Part model, mm, in its own coordinate system. A direction names the side the tool comes from. Give positions to 0.01 mm unless a question says otherwise; leave off trailing zeros. Write each loop counter-clockwise with the first axis right and the second up, starting at its lowest first coordinate (ties: lowest second). Pieces come first, ordered by that corner, then holes. Notation, with made-up numbers: M -7.75,8.25 L 25.25,8.25 A33 cw 25.25,47.25 Z; hole C 85,86.25 d2. An arc over 180 degrees is marked long. Answer as CSV lines item,"result". Start each with the question number.
1) Pin check, flat tips, straight feed: pin 1 Ø4 at (y, z) = (-3.5, -1.5) entering from -X; pin 2 Ø5 at (x, z) = (6.5, -7.5) entering from -Y; pin 3 Ø2 at (x, z) = (9, 8.5) entering from -Y. Stop position of each tip, or through.
2) Slice it at A-A, the plane y = 0. Give the cut face in (x, z), plus the area to 3 significant figures.
3) Slice it at B-B, the plane x = 0. Give the cut face in (y, z).
4) Wall check: line 1 along Y through (x, z) = (0, 2); line 2 along Y through (x, z) = (-0.75, 4); line 3 along X through (y, z) = (-6.25, -12.5). Give the ranges that are in metal, low to high. Write a range as from..to.
5) Mould opens along X. For faces 3 (the cylindrical face through (-11.34, 6.56, 0.22)), 4 (the cylindrical face through (-6.29, 10.918, 0.217)), 5 (the cylindrical face through (7.7, -10.6, 0.2)) say: pulls with the +X half, pulls with the -X half, needs draft (parallel to the pull), parting line crosses it, or undercut.
6) Tool access for faces 1 (the cylindrical face through (-2.73, -12.812, 0.217)), 2 (the cylindrical face through (8.44, 9.356, 0.217)): list every direction of +Z, -Z, +X, -X, +Y, -Y with a clear straight run to the whole face (end or side of a thin tool).
```python
from build123d import *

# Parameters (mm, degrees)
F0_R     = 12.5
F1_DEPTH = 15.5
F0_R_2   = 11.1
F2_DEPTH = 15.5


with BuildPart() as f1:
    # F0 (on Top) → F1 (new body, symmetric)
    with BuildSketch(Plane.XY):
        with BuildLine():
            Line((0.5, -13.090455), (0.480916, -12.590819))
            ThreePointArc((0.480916, -12.590819), (1.317059, -12.530976), (2.147372, -12.415667))
            Line((2.147372, -12.415667), (2.232585, -12.908353))
            ThreePointArc((2.232585, -12.908353), (2.723643, -12.813734), (3.210732, -12.700441))
            Line((3.210732, -12.700441), (3.088185, -12.215691))
            ThreePointArc((3.088185, -12.215691), (3.893614, -11.983312), (4.681809, -11.697892))
            Line((4.681809, -11.697892), (4.867595, -12.162094))
            ThreePointArc((4.867595, -12.162094), (5.32825, -11.967445), (5.78114, -11.755357))
            Line((5.78114, -11.755357), (5.560486, -11.306679))
            ThreePointArc((5.560486, -11.306679), (6.3, -10.91192), (7.011628, -10.468862))
            Line((7.011628, -10.468862), (7.289868, -10.884293))
            ThreePointArc((7.289868, -10.884293), (7.699987, -10.598123), (8.098885, -10.296508))
            Line((8.098885, -10.296508), (7.789767, -9.903511))
            ThreePointArc((7.789767, -9.903511), (8.431046, -9.363625), (9.035006, -8.782293))
            Line((9.035006, -8.782293), (9.393538, -9.130796))
            ThreePointArc((9.393538, -9.130796), (9.735197, -8.765611), (10.062669, -8.387651))
            Line((10.062669, -8.387651), (9.678598, -8.067512))
            ThreePointArc((9.678598, -8.067512), (10.193614, -7.406094), (10.663511, -6.711895))
            Line((10.663511, -6.711895), (11.086666, -6.97824))
            ThreePointArc((11.086666, -6.97824), (11.344933, -6.55), (11.586666, -6.112215))
            Line((11.586666, -6.112215), (11.144427, -5.878924))
            ThreePointArc((11.144427, -5.878924), (11.510673, -5.124882), (11.825969, -4.348155))
            Line((11.825969, -4.348155), (12.295254, -4.520701))
            ThreePointArc((12.295254, -4.520701), (12.45884, -4.048123), (12.604271, -3.569645))
            Line((12.604271, -3.569645), (12.123192, -3.433399))
            ThreePointArc((12.123192, -3.433399), (12.32466, -2.619687), (12.471576, -1.79438))
            Line((12.471576, -1.79438), (12.966479, -1.865586))
            ThreePointArc((12.966479, -1.865586), (13.028237, -1.369323), (13.071008, -0.871064))
            Line((13.071008, -0.871064), (12.572114, -0.837817))
            ThreePointArc((12.572114, -0.837817), (12.6, 0), (12.572114, 0.837817))
            Line((12.572114, 0.837817), (13.071008, 0.871064))
            ThreePointArc((13.071008, 0.871064), (13.028237, 1.369323), (12.966479, 1.865586))
            Line((12.966479, 1.865586), (12.471576, 1.79438))
            ThreePointArc((12.471576, 1.79438), (12.32466, 2.619687), (12.123192, 3.433399))
            Line((12.123192, 3.433399), (12.604271, 3.569645))
            ThreePointArc((12.604271, 3.569645), (12.45884, 4.048123), (12.295254, 4.520701))
            Line((12.295254, 4.520701), (11.825969, 4.348155))
            ThreePointArc((11.825969, 4.348155), (11.510673, 5.124882), (11.144427, 5.878924))
            Line((11.144427, 5.878924), (11.586666, 6.112215))
            ThreePointArc((11.586666, 6.112215), (11.344933, 6.55), (11.086666, 6.97824))
            Line((11.086666, 6.97824), (10.663511, 6.711895))
            ThreePointArc((10.663511, 6.711895), (10.193614, 7.406094), (9.678598, 8.067512))
            Line((9.678598, 8.067512), (10.062669, 8.387651))
            ThreePointArc((10.062669, 8.387651), (9.735197, 8.765611), (9.393538, 9.130796))
            Line((9.393538, 9.130796), (9.035006, 8.782293))
            ThreePointArc((9.035006, 8.782293), (8.431046, 9.363625), (7.789767, 9.903511))
            Line((7.789767, 9.903511), (8.098885, 10.296508))
            ThreePointArc((8.098885, 10.296508), (7.699987, 10.598123), (7.289868, 10.884293))
            Line((7.289868, 10.884293), (7.011628, 10.468862))
            ThreePointArc((7.011628, 10.468862), (6.3, 10.91192), (5.560486, 11.306679))
            Line((5.560486, 11.306679), (5.78114, 11.755357))
            ThreePointArc((5.78114, 11.755357), (5.32825, 11.967445), (4.867595, 12.162094))
            Line((4.867595, 12.162094), (4.681809, 11.697892))
            ThreePointArc((4.681809, 11.697892), (3.893614, 11.983312), (3.088185, 12.215691))
            Line((3.088185, 12.215691), (3.210732, 12.700441))
            ThreePointArc((3.210732, 12.700441), (2.723643, 12.813734), (2.232585, 12.908353))
            Line((2.232585, 12.908353), (2.147372, 12.415667))
            ThreePointArc((2.147372, 12.415667), (1.317059, 12.530976), (0.480916, 12.590819))
            Line((0.480916, 12.590819), (0.5, 13.090455))
            ThreePointArc((0.5, 13.090455), (0, 13.1), (-0.5, 13.090455))
            Line((-0.5, 13.090455), (-0.480916, 12.590819))
            ThreePointArc((-0.480916, 12.590819), (-1.317059, 12.530976), (-2.147372, 12.415667))
            Line((-2.147372, 12.415667), (-2.232585, 12.908353))
            ThreePointArc((-2.232585, 12.908353), (-2.723643, 12.813734), (-3.210732, 12.700441))
            Line((-3.210732, 12.700441), (-3.088185, 12.215691))
            ThreePointArc((-3.088185, 12.215691), (-3.893614, 11.983312), (-4.681809, 11.697892))
            Line((-4.681809, 11.697892), (-4.867595, 12.162094))
            ThreePointArc((-4.867595, 12.162094), (-5.32825, 11.967445), (-5.78114, 11.755357))
            Line((-5.78114, 11.755357), (-5.560486, 11.306679))
            ThreePointArc((-5.560486, 11.306679), (-6.3, 10.91192), (-7.011628, 10.468862))
            Line((-7.011628, 10.468862), (-7.289868, 10.884293))
            ThreePointArc((-7.289868, 10.884293), (-7.699987, 10.598123), (-8.098885, 10.296508))
            Line((-8.098885, 10.296508), (-7.789767, 9.903511))
            ThreePointArc((-7.789767, 9.903511), (-8.431046, 9.363625), (-9.035006, 8.782293))
            Line((-9.035006, 8.782293), (-9.393538, 9.130796))
            ThreePointArc((-9.393538, 9.130796), (-9.735197, 8.765611), (-10.062669, 8.387651))
            Line((-10.062669, 8.387651), (-9.678598, 8.067512))
            ThreePointArc((-9.678598, 8.067512), (-10.193614, 7.406094), (-10.663511, 6.711895))
            Line((-10.663511, 6.711895), (-11.086666, 6.97824))
            ThreePointArc((-11.086666, 6.97824), (-11.344933, 6.55), (-11.586666, 6.112215))
            Line((-11.586666, 6.112215), (-11.144427, 5.878924))
            ThreePointArc((-11.144427, 5.878924), (-11.510673, 5.124882), (-11.825969, 4.348155))
            Line((-11.825969, 4.348155), (-12.295254, 4.520701))
            ThreePointArc((-12.295254, 4.520701), (-12.45884, 4.048123), (-12.604271, 3.569645))
            Line((-12.604271, 3.569645), (-12.123192, 3.433399))
            ThreePointArc((-12.123192, 3.433399), (-12.32466, 2.619687), (-12.471576, 1.79438))
            Line((-12.471576, 1.79438), (-12.966479, 1.865586))
            ThreePointArc((-12.966479, 1.865586), (-13.028237, 1.369323), (-13.071008, 0.871064))
            Line((-13.071008, 0.871064), (-12.572114, 0.837817))
            ThreePointArc((-12.572114, 0.837817), (-12.6, 0), (-12.572114, -0.837817))
            Line((-12.572114, -0.837817), (-13.071008, -0.871064))
            ThreePointArc((-13.071008, -0.871064), (-13.028237, -1.369323), (-12.966479, -1.865586))
            Line((-12.966479, -1.865586), (-12.471576, -1.79438))
            ThreePointArc((-12.471576, -1.79438), (-12.32466, -2.619687), (-12.123192, -3.433399))
            Line((-12.123192, -3.433399), (-12.604271, -3.569645))
            ThreePointArc((-12.604271, -3.569645), (-12.45884, -4.048123), (-12.295254, -4.520701))
            Line((-12.295254, -4.520701), (-11.825969, -4.348155))
            ThreePointArc((-11.825969, -4.348155), (-11.510673, -5.124882), (-11.144427, -5.878924))
            Line((-11.144427, -5.878924), (-11.586666, -6.112215))
            ThreePointArc((-11.586666, -6.112215), (-11.344933, -6.55), (-11.086666, -6.97824))
            Line((-11.086666, -6.97824), (-10.663511, -6.711895))
            ThreePointArc((-10.663511, -6.711895), (-10.193614, -7.406094), (-9.678598, -8.067512))
            Line((-9.678598, -8.067512), (-10.062669, -8.387651))
            ThreePointArc((-10.062669, -8.387651), (-9.735197, -8.765611), (-9.393538, -9.130796))
            Line((-9.393538, -9.130796), (-9.035006, -8.782293))
            ThreePointArc((-9.035006, -8.782293), (-8.431046, -9.363625), (-7.789767, -9.903511))
            Line((-7.789767, -9.903511), (-8.098885, -10.296508))
            ThreePointArc((-8.098885, -10.296508), (-7.699987, -10.598123), (-7.289868, -10.884293))
            Line((-7.289868, -10.884293), (-7.011628, -10.468862))
            ThreePointArc((-7.011628, -10.468862), (-6.3, -10.91192), (-5.560486, -11.306679))
            Line((-5.560486, -11.306679), (-5.78114, -11.755357))
            ThreePointArc((-5.78114, -11.755357), (-5.32825, -11.967445), (-4.867595, -12.162094))
            Line((-4.867595, -12.162094), (-4.681809, -11.697892))
            ThreePointArc((-4.681809, -11.697892), (-3.893614, -11.983312), (-3.088185, -12.215691))
            Line((-3.088185, -12.215691), (-3.210732, -12.700441))
            ThreePointArc((-3.210732, -12.700441), (-2.723643, -12.813734), (-2.232585, -12.908353))
            Line((-2.232585, -12.908353), (-2.147372, -12.415667))
            ThreePointArc((-2.147372, -12.415667), (-1.317059, -12.530976), (-0.480916, -12.590819))
            Line((-0.480916, -12.590819), (-0.5, -13.090455))
            ThreePointArc((-0.5, -13.090455), (0, -13.1), (0.5, -13.090455))
        make_face()
        Circle(F0_R, mode=Mode.SUBTRACT)
    extrude(amount=F1_DEPTH, both=True)

    # F0 (on Top) → F2 (join, symmetric)
    with BuildSketch(Plane.XY):
        Circle(F0_R)
        Circle(F0_R_2, mode=Mode.SUBTRACT)
    extrude(amount=F2_DEPTH, both=True)


solid = f1.part
```
Found:
1,pin 1,"x = -13.01"
1,pin 2,"y = -12.16"
1,pin 3,"y = -10.37"
2,outline,"M -12.6,-15.5 L -11.1,-15.5 L -11.1,15.5 L -12.6,15.5 Z; M 11.1,-15.5 L 12.6,-15.5 L 12.6,15.5 L 11.1,15.5 Z"
2,area,"93.0 mm²"
3,outline,"M -13.1,-15.5 L -11.1,-15.5 L -11.1,15.5 L -13.1,15.5 Z; M 11.1,-15.5 L 13.1,-15.5 L 13.1,15.5 L 11.1,15.5 Z"
4,line 1,"-13.1..-11.1, 11.1..13.1"
4,line 2,"-12.58..-11.07, 11.07..12.58"
4,line 3,"-11.51..-9.17, 9.17..11.51"
5,face 3,"pulls with the -X half"
5,face 4,"undercut"
5,face 5,"pulls with the +X half"
6,face 1,"+Z, -Z, -X, -Y"
6,face 2,"+Z, -Z"
